Here's how the part is built. I have some questions about the finished solid (model axes, mm). Face numbers are marked on the shaded views. Round coordinates to 2 decimals unless told otherwise and drop trailing zeros. Write each loop counter-clockwise with the first axis right and the second up, starting at its lowest first coordinate (ties: lowest second). Pieces come first, ordered by that corner, then holes. Notation, with made-up numbers: (27, 8) - (69, 8) arc R22 ccw to (69, 21) - close; hole circle Ø5 at (-16.5, 26). An arc over 180 degrees is marked (long way). One line per item, written item: value. Start each with the question number.
Item 1: Thinking about a two-plate mould opening in Z: for the marked faces 1, 2 and 3, which applies, released by +Z, released by -Z, zero draft, split by the parting line, or undercut?
Item 2: If I drill on line 1 (Z direction, x = -44.5, y = -37); line 2 (Y direction, x = -52.5, z = 5.75) (3 decimals); line 3 (X direction, y = -32, z = 277), over which ranges is the centre line in solid material (lowest first)?
Item 3: For P1, Ø8, axis at x = -182, y = 72.5, coming from the -Z side; P2, Ø5, axis at x = -53, y = -32.5, coming from the +Z side; P3, Ø4, axis at x = -135.5, z = 60.5, coming from the +Y side, each with a flat end and sliding along its axis, tell me the tip position at first contact or that it passes through.
Item 4: Imagine slicing it at A-A, the plane z = 57. Please give me the cut outline in (x, y), then the cut area to 3 significant figures.
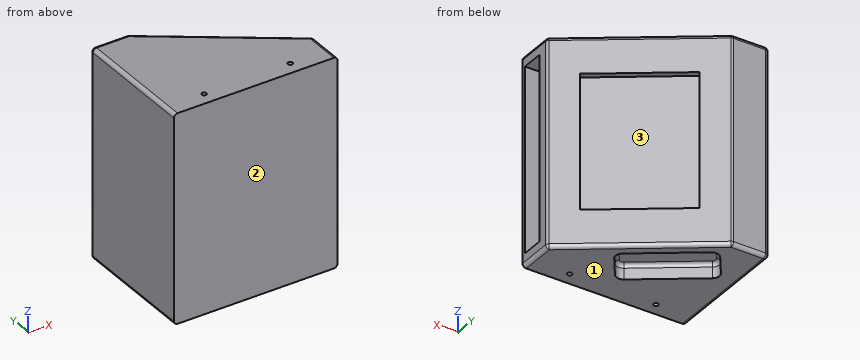
```python
from build123d import *

# Parameters (mm, degrees)
SKETCH1_W           = 50
SKETCH1_H           = 170.451051634
BOSS_EXTRUDE1_DEPTH = 282
CUT_EXTRUDE1_DEPTH  = 8
SKETCH5_R           = 3.175
CUT_EXTRUDE3_DEPTH  = 7.7
SKETCH6_R           = 3.175
CUT_EXTRUDE4_DEPTH  = 7.7
FILLET4_R           = 5
SKETCH7_W           = 250
SKETCH7_H           = 30
CUT_EXTRUDE6_DEPTH  = 150
CUT_EXTRUDE7_DEPTH  = 20
FILLET5_R           = 10
FILLET6_R           = 5


with BuildPart() as part:
    # Sketch1 → Boss-Extrude1 (new body)
    with BuildSketch(Plane.XY):
        with Locations((-197.021929301, 35.225525817)):
            Rectangle(SKETCH1_W, SKETCH1_H)
        Polygon((0, -50), (0, 0), (-172.021929301, 120.451051634), (-172.021929301, -50), align=None)
    extrude(amount=BOSS_EXTRUDE1_DEPTH)

    # Sketch3 → Cut-Extrude1 (cut)
    with BuildSketch(Plane(origin=(0, 0, 0), x_dir=(0.819152044, -0.573576436, 0), z_dir=(0.573576436, 0.819152044, 0))):
        Polygon((-37.234042553, -232), (-172.765957447, -50), (-172.765957447, -232), align=None)
        Polygon((-37.234042553, -50), (-172.765957447, -50), (-37.234042553, -232), align=None)
    extrude(amount=-CUT_EXTRUDE1_DEPTH, mode=Mode.SUBTRACT)

    # Sketch5 → Cut-Extrude3 (cut)
    with BuildSketch(Plane.XY.offset(282)):
        with Locations((-52.5, -32.5)):
            Circle(SKETCH5_R)
        with Locations((-169.521929301, -32.5)):
            Circle(SKETCH5_R)
    extrude(amount=-CUT_EXTRUDE3_DEPTH, mode=Mode.SUBTRACT)

    # Sketch6 → Cut-Extrude4 (cut)
    with BuildSketch(Plane(origin=(0, 0, 0), x_dir=(-1, 0, 0), z_dir=(0, 0, -1))):
        with Locations((169.521929301, -32.5)):
            Circle(SKETCH6_R)
        with Locations((52.5, -32.5)):
            Circle(SKETCH6_R)
    extrude(amount=-CUT_EXTRUDE4_DEPTH, mode=Mode.SUBTRACT)

    # Fillet4
    fillet4_edges = [part.edges().sort_by_distance(p)[0] for p in [
        (-222.021929301, 35.225525817, 282),
        (-172.021929301, 120.451051634, 141),
        (0, 0, 141),
        (-222.021929301, 120.451051634, 141),
        (0, -25, 282),
        (-86.01096465, 60.225525817, 282),
        (-197.021929301, 120.451051634, 282),
        (-86.01096465, 60.225525817, 0),
        (0, -25, 0),
        (-222.021929301, 35.225525817, 0),
        (-197.021929301, 120.451051634, 0),
    ]]
    fillet(fillet4_edges, radius=FILLET4_R)

    # Sketch7 → Cut-Extrude6 (cut)
    with BuildSketch(Plane(origin=(0, 0, 0), x_dir=(0, 0, -1), z_dir=(1, 0, 0))):
        with Locations((-141, -30)):
            Rectangle(SKETCH7_W, SKETCH7_H)
    extrude(amount=-CUT_EXTRUDE6_DEPTH, mode=Mode.SUBTRACT)

    # Sketch9 → Cut-Extrude7 (cut)
    with BuildSketch(Plane(origin=(0, 0, 0), x_dir=(-1, 0, 0), z_dir=(0, 0, -1))):
        Polygon((200.305363971, 54.801104583), (102.007118657, -14.028067779), (70.460414657, 31.025294657), (168.758659972, 99.854467019), align=None)
    extrude(amount=-CUT_EXTRUDE7_DEPTH, mode=Mode.SUBTRACT)

    # Fillet5
    fillet5_edges = [part.edges().sort_by_distance(p)[0] for p in [
        (-200.305363971, 54.801104583, 10),
        (-102.007118657, -14.028067779, 10),
        (-70.460414657, 31.025294657, 10),
        (-168.758659972, 99.854467019, 10),
    ]]
    fillet(fillet5_edges, radius=FILLET5_R)

    # Fillet6
    fillet6_edges = [part.edges().sort_by_distance(p)[0] for p in [
        (-86.233766657, 8.498613439, 20),
        (-119.609537315, 65.439880838, 20),
        (-151.156241314, 20.386518402, 20),
        (-184.532011972, 77.327785801, 20),
        (-196.226156695, 55.520378886, 20),
        (-168.039385669, 95.775259743, 20),
        (-102.726392959, -9.948860503, 20),
        (-74.539621934, 30.306020354, 20),
    ]]
    fillet(fillet6_edges, radius=FILLET6_R)


solid = part.part
```
Values follow:
1. face 1: released by -Z
1. face 2: zero draft
1. face 3: undercut
2. line 1: z = 0 to 16, 266 to 282
2. line 2: y = -50 to -35.675, -29.325 to 36.761
2. line 3: x = -222.02 to -172.66, -166.39 to -55.64, -49.36 to 0
3. P1: stops at z = 17.78
3. P2: stops at z = 274.3
3. P3: stops at y = 86.51
4. outline: (-222.02, -50) - (0, -50) - (0, -45) - (-150, -45) - (-150, -15) - (0, -15) - (0, -2.6) arc R5 ccw to (-2.13, 1.49) - (-30.5, 21.36) - (-35.09, 14.8) - (-146.11, 92.54) - (-141.52, 99.09) - (-170.73, 119.55) arc R5 ccw to (-173.6, 120.45) - (-217.02, 120.45) arc R5 ccw to (-222.02, 115.45) - close
4. area: 21,900 mm^2
